Check sheet for the drawn part. Datum: minimum x, y, z corner. Units: mm. Round coordinates to 2 decimals unless told otherwise and drop trailing zeros. Order: outer loops, then holes, each group sorted by start corner. A loop starts at its lowest first (then second) coordinate and runs counter-clockwise, first axis right, second up. Notation, with made-up numbers: M -29.5,66.25 L -3.5,66.25 A15 cw -3.5,76.25 Z; hole C -24.5,86.5 d11. An arc over 180 degrees is marked long. Use one line per item in the form item = value. Start each with the question number.
Item 1: Cross-section at B-B on x = 17.5. Enter the section's corners in (y, z).
Item 2: Thickness scan on probe 1 along X at (y, z) = (2.05, 57); probe 2 along Z at (x, y) = (26.25, 1); probe 3 along Z at (x, y) = (18, 1.35). Record the ranges inside material, lowest first. Write a range as [from, to].
Item 3: Cross-section at C-C on y = 0.5. Enter the section's corners in (x, z).
Item 4: Cross-section at D-D on z = 48.5. Enter the section's corners in (x, y).
Item 5: Cross-section at A-A on z = 57. Enter the section's corners in (x, y).
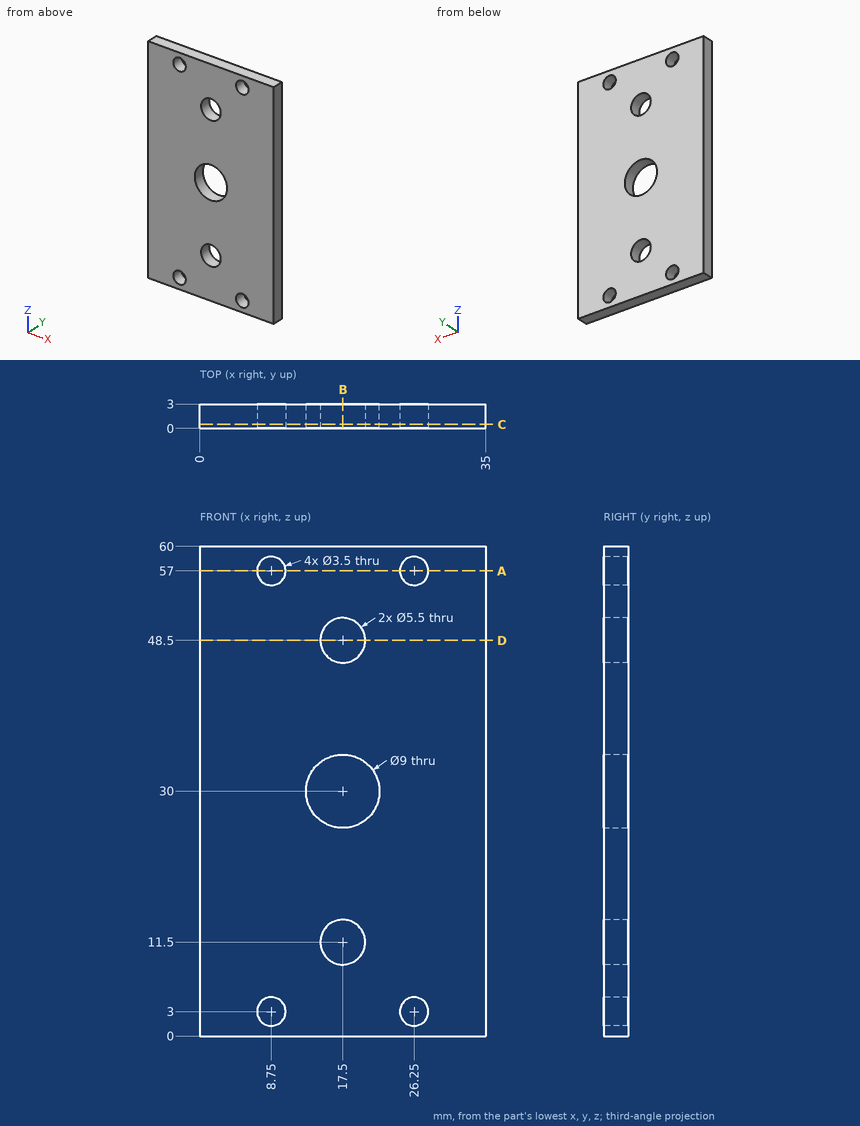
Output values:
q1.outline = M 0,0 L 3,0 L 3,8.75 L 0,8.75 Z; M 0,14.25 L 3,14.25 L 3,25.5 L 0,25.5 Z; M 0,34.5 L 3,34.5 L 3,45.75 L 0,45.75 Z; M 0,51.25 L 3,51.25 L 3,60 L 0,60 Z
q2.probe_1 = [0, 7], [10.5, 24.5], [28, 35]
q2.probe_2 = [0, 1.25], [4.75, 55.25], [58.75, 60]
q2.probe_3 = [0, 8.8], [14.2, 25.53], [34.47, 45.8], [51.2, 60]
q3.outline = M 0,0 L 35,0 L 35,60 L 0,60 Z; hole C 8.75,3 d3.5; hole C 8.75,57 d3.5; hole C 17.5,30 d9; hole C 17.5,11.5 d5.5; hole C 17.5,48.5 d5.5; hole C 26.25,3 d3.5; hole C 26.25,57 d3.5
q4.outline = M 0,0 L 14.75,0 L 14.75,3 L 0,3 Z; M 20.25,0 L 35,0 L 35,3 L 20.25,3 Z
q5.outline = M 0,0 L 7,0 L 7,3 L 0,3 Z; M 10.5,0 L 24.5,0 L 24.5,3 L 10.5,3 Z; M 28,0 L 35,0 L 35,3 L 28,3 Z
